from build123d import *

# Parameters (mm, degrees)
F0_R     = 1.5
F1_DEPTH = 3
F2_W     = 81
F2_H     = 3
F3_DEPTH = 30
F5_DEPTH = 3


with BuildPart() as f1:
    # F0 (on Top) → F1 (new body)
    with BuildSketch(Plane.XY):
        with BuildLine():
            Line((81, 11.4), (0, 11.4))
            Line((0, 11.4), (0, 0))
            Line((0, 0), (0, -12))
            ThreePointArc((0, -12), (0.87868, -14.12132), (3, -15))
            Line((3, -15), (12, -15))
            ThreePointArc((12, -15), (14.12132, -14.12132), (15, -12))
            Line((15, -12), (15, -3))
            ThreePointArc((15, -3), (15.87868, -0.87868), (18, 0))
            Line((18, 0), (63, 0))
            ThreePointArc((63, 0), (65.12132, -0.87868), (66, -3))
            Line((66, -3), (66, -12))
            ThreePointArc((66, -12), (66.87868, -14.12132), (69, -15))
            Line((69, -15), (78, -15))
            ThreePointArc((78, -15), (80.12132, -14.12132), (81, -12))
            Line((81, -12), (81, 0))
            Line((81, 0), (81, 11.4))
        make_face()
        with Locations((5, 5)):
            Circle(F0_R, mode=Mode.SUBTRACT)
        with Locations((76, 5)):
            Circle(F0_R, mode=Mode.SUBTRACT)
    extrude(amount=F1_DEPTH)

    # F2 (on face) → F3 (join)
    with BuildSketch(Plane.XY.offset(3)):
        with Locations((40.5, 9.9)):
            Rectangle(F2_W, F2_H)
    extrude(amount=F3_DEPTH)

    # F4 (on face) → F5 (cut, through all)
    with BuildSketch(Plane.XZ.offset(-8.4)):
        with BuildLine():
            Line((72, 33), (9, 33))
            Line((9, 33), (9, 15))
            Line((9, 15), (22, 15))
            ThreePointArc((22, 15), (24.12132, 14.12132), (25, 12))
            Line((25, 12), (25, 8))
            Line((25, 8), (56, 8))
            Line((56, 8), (56, 12))
            ThreePointArc((56, 12), (56.87868, 14.12132), (59, 15))
            Line((59, 15), (72, 15))
            Line((72, 15), (72, 33))
        make_face()
    extrude(amount=-F5_DEPTH, mode=Mode.SUBTRACT)


solid = f1.part
For this review, take the finished solid that the model builds, in its own axes (mm). A direction names the side the tool comes from. Coordinates: 2 decimals unless noted, no trailing zeros. Order: outer loops, then holes, each group sorted by start corner. A loop starts at its lowest first (then second) coordinate and runs counter-clockwise, first axis right, second up. Notation, with made-up numbers: (89.25, 25) -> (103.25, 25) arc R35 ccw to (103.25, 60) -> close; hole circle Ø8 at (54, 39). An arc over 180 degrees is marked (long way). Return JSON: item names as keys, results as strings.
1. We need section B-B on z = 30.5. Write out the cut boundary in (x, y).
Answer block:
{"outline": "(0, 8.4) -> (9, 8.4) -> (9, 11.4) -> (0, 11.4) -> close; (72, 8.4) -> (81, 8.4) -> (81, 11.4) -> (72, 11.4) -> close"}
2. For pin 1 Ø10 at (x, y) = (63, 3.5) entering from +Z; pin 2 Ø3 at (y, z) = (6.5, 8) entering from +X; pin 3 Ø3.5 at (x, z) = (33, 1) entering from -Y; pin 4 Ø0.9 at (x, y) = (45.5, 10) entering from +Z, all flat-tipped, find the tip position at first contact; note any pin that passes through.
Answer block:
{"pin 1": "z = 15", "pin 2": "through", "pin 3": "y = 0", "pin 4": "z = 8"}
3. The part is to be moulded in two halves that separate along X. For faces 1 (the flat face through (40, 1, 0)), 2 (the flat face through (0, 9, 10)), 3 (the flat face through (25, 10, 10)), 4 (the flat face through (65, 10, 15)), say which applies: +X half, -X half, draft (parallel to the pull), parting line (faces both ways), or undercut.
Answer block:
{"face 1": "draft", "face 2": "-X half", "face 3": "undercut", "face 4": "undercut"}
4. We need section A-A on x = 76. Write out the cut boundary in (y, z), and give its area (3 significant figures).
Answer block:
{"outline": "(-15, 0) -> (3.5, 0) -> (3.5, 3) -> (-15, 3) -> close; (6.5, 0) -> (11.4, 0) -> (11.4, 33) -> (8.4, 33) -> (8.4, 3) -> (6.5, 3) -> close", "area": "160 mm²"}
5. We need section D-D on y = -7.75. Write out the cut boundary in (x, z), and give its area (3 significant figures).
Answer block:
{"outline": "(0, 0) -> (15, 0) -> (15, 3) -> (0, 3) -> close; (66, 0) -> (81, 0) -> (81, 3) -> (66, 3) -> close", "area": "90.0 mm²"}
6. For line 1 (Y direction, x = 5, z = 1); line 2 (Z direction, x = 74, y = -9.25); line 3 (Y direction, x = 77, z = 18.5), list the stretches that pass through material, from the lowest coordinate up. Write a range as from..to.
Answer block:
{"line 1": "-15..3.5, 6.5..11.4", "line 2": "0..3", "line 3": "8.4..11.4"}
7. We need section C-C on y = 5. Write out the cut boundary in (x, z).
Answer block:
{"outline": "(0, 0) -> (3.5, 0) -> (3.5, 3) -> (0, 3) -> close; (6.5, 0) -> (74.5, 0) -> (74.5, 3) -> (6.5, 3) -> close; (77.5, 0) -> (81, 0) -> (81, 3) -> (77.5, 3) -> close"}
8. Machinability: for faces 5 (the flat face through (66, -7, 1)), 6 (the flat face through (40, 2, 3)), 7 (the flat face through (7, -15, 1)), 8 (the flat face through (40, 10, 8)), which of the approach directions +Z, -Z, +X, -X, +Y, -Y give a long, thin tool a straight path to every point of the face, cutting with its end or side? Answer none if there is none.
Answer block:
{"face 5": "+Z, -Z, -Y", "face 6": "+Z, +X, -X, -Y", "face 7": "+Z, -Z, +X, -X, -Y", "face 8": "+Z, +Y, -Y"}
